from build123d import *

# Parameters (mm, degrees)
SKETCH1_R           = 2.5
BOSS_EXTRUDE1_DEPTH = 147


with BuildPart() as part:
    # Sketch1 → Boss-Extrude1 (new body)
    with BuildSketch(Plane(origin=(0, 0, 0), x_dir=(1, 0, 0), z_dir=(0, 1, 0))):
        with BuildLine():
            Line((3.9, 10), (8.5, 10))
            ThreePointArc((8.5, 10), (9.560660172, 9.560660172), (10, 8.5))
            Line((10, 8.5), (10, 3.9))
            Line((10, 3.9), (9.2, 3.9))
            Line((9.2, 3.9), (9.2, 3.1))
            Line((9.2, 3.1), (8.2, 3.1))
            Line((8.2, 3.1), (8.2, 5.5))
            Line((8.2, 5.5), (6.77, 5.5))
            Line((6.77, 5.5), (3.9, 2.63))
            Line((3.9, 2.63), (3.9, 0))
            Line((3.9, 0), (3.9, -2.63))
            Line((3.9, -2.63), (6.77, -5.5))
            Line((6.77, -5.5), (8.2, -5.5))
            Line((8.2, -5.5), (8.2, -3.1))
            Line((8.2, -3.1), (9.2, -3.1))
            Line((9.2, -3.1), (9.2, -3.9))
            Line((9.2, -3.9), (10, -3.9))
            Line((10, -3.9), (10, -8.5))
            ThreePointArc((10, -8.5), (9.560660172, -9.560660172), (8.5, -10))
            Line((8.5, -10), (3.9, -10))
            Line((3.9, -10), (3.9, -9.2))
            Line((3.9, -9.2), (3.1, -9.2))
            Line((3.1, -9.2), (3.1, -8.2))
            Line((3.1, -8.2), (5.5, -8.2))
            Line((5.5, -8.2), (5.5, -6.77))
            Line((5.5, -6.77), (2.63, -3.9))
            Line((2.63, -3.9), (0, -3.9))
            Line((0, -3.9), (-2.63, -3.9))
            Line((-2.63, -3.9), (-5.5, -6.77))
            Line((-5.5, -6.77), (-5.5, -8.2))
            Line((-5.5, -8.2), (-3.1, -8.2))
            Line((-3.1, -8.2), (-3.1, -9.2))
            Line((-3.1, -9.2), (-3.9, -9.2))
            Line((-3.9, -9.2), (-3.9, -10))
            Line((-3.9, -10), (-8.5, -10))
            ThreePointArc((-8.5, -10), (-9.560660172, -9.560660172), (-10, -8.5))
            Line((-10, -8.5), (-10, -3.9))
            Line((-10, -3.9), (-9.2, -3.9))
            Line((-9.2, -3.9), (-9.2, -3.1))
            Line((-9.2, -3.1), (-8.2, -3.1))
            Line((-8.2, -3.1), (-8.2, -5.5))
            Line((-8.2, -5.5), (-6.77, -5.5))
            Line((-6.77, -5.5), (-3.9, -2.63))
            Line((-3.9, -2.63), (-3.9, 0))
            Line((-3.9, 0), (-3.9, 2.63))
            Line((-3.9, 2.63), (-6.77, 5.5))
            Line((-6.77, 5.5), (-8.2, 5.5))
            Line((-8.2, 5.5), (-8.2, 3.1))
            Line((-8.2, 3.1), (-9.2, 3.1))
            Line((-9.2, 3.1), (-9.2, 3.9))
            Line((-9.2, 3.9), (-10, 3.9))
            Line((-10, 3.9), (-10, 8.5))
            ThreePointArc((-10, 8.5), (-9.560660172, 9.560660172), (-8.5, 10))
            Line((-8.5, 10), (-3.9, 10))
            Line((-3.9, 10), (-3.9, 9.2))
            Line((-3.9, 9.2), (-3.1, 9.2))
            Line((-3.1, 9.2), (-3.1, 8.2))
            Line((-3.1, 8.2), (-5.5, 8.2))
            Line((-5.5, 8.2), (-5.5, 6.77))
            Line((-5.5, 6.77), (-2.63, 3.9))
            Line((-2.63, 3.9), (2.63, 3.9))
            Line((2.63, 3.9), (5.5, 6.77))
            Line((5.5, 6.77), (5.5, 8.2))
            Line((5.5, 8.2), (3.1, 8.2))
            Line((3.1, 8.2), (3.1, 9.2))
            Line((3.1, 9.2), (3.9, 9.2))
            Line((3.9, 9.2), (3.9, 10))
        make_face()
        Circle(SKETCH1_R, mode=Mode.SUBTRACT)
    extrude(amount=BOSS_EXTRUDE1_DEPTH)


solid = part.part
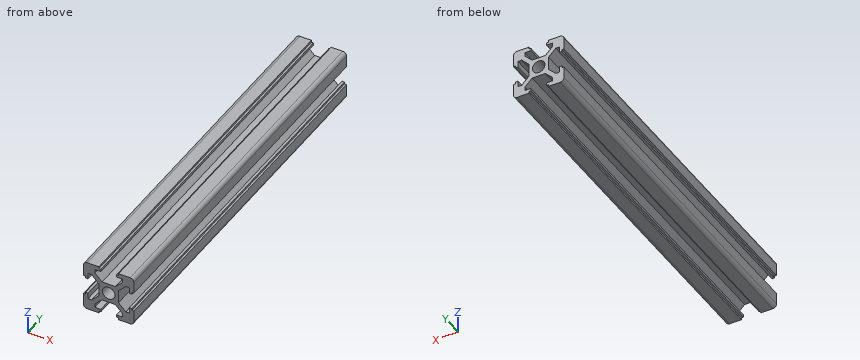
Build history of the part. All positions in model axes, mm. Give positions to 0.01 mm unless a question says otherwise; leave off trailing zeros. Order: outer loops, then holes, each group sorted by start corner. A loop starts at its lowest first (then second) coordinate and runs counter-clockwise, first axis right, second up. Notation, with made-up numbers: M 25,47 L 53,47 A25 cw 53,70 Z; hole C 62.25,-37.75 d4. An arc over 180 degrees is marked long. Put each result on its own line as item: value.
Item 1: Cut at A-A on x = 0. Write the cut outline in (y, z), then the cut area to 3 significant figures.
Results are:
outline: M 0,-3.9 L 147,-3.9 L 147,-2.5 L 0,-2.5 Z; M 0,2.5 L 147,2.5 L 147,3.9 L 0,3.9 Z
area: 412 mm2
Item 2: Drop flat-ended pins along their axis: pin 1 Ø0.6 at (y, z) = (100, -3.5) entering from +X; pin 2 Ø4 at (y, z) = (95, 1) entering from -X; pin 3 Ø0.8 at (y, z) = (103, -9) entering from +X. Give the stop position or say it passes through.
Results are:
pin 1: x = 9.2
pin 2: x = -4.27
pin 3: x = 10
Item 3: Cut at B-B on z = 0. Write the cut outline in (x, y), then the cut area to 3 significant figures.
Results are:
outline: M -3.9,0 L -2.5,0 L -2.5,147 L -3.9,147 Z; M 2.5,0 L 3.9,0 L 3.9,147 L 2.5,147 Z
area: 412 mm2
Item 4: Wall check: probe 1 along X at (y, z) = (112, 8); probe 2 along Z at (x, y) = (0, 38). Give the ranges that are in metal, low to high.
Results are:
probe 1: -10 to -5.5, 5.5 to 10
probe 2: -3.9 to -2.5, 2.5 to 3.9
